Build history of the part. All positions in model axes, mm. A direction names the side the tool comes from. Coordinates: 2 decimals unless noted, no trailing zeros. Order: outer loops, then holes, each group sorted by start corner. A loop starts at its lowest first (then second) coordinate and runs counter-clockwise, first axis right, second up. Notation, with made-up numbers: (3, 84.5) - (37, 84.5) arc R15 ccw to (37, 111.5) - close; hole circle Ø11 at (80, -33.75). An arc over 180 degrees is marked (long way). Return JSON: item names as keys, results as strings.
from build123d import *

# Parameters (mm, degrees)
BOSS_EXTRUDE1_DEPTH = 5
CUT_EXTRUDE1_DEPTH  = 8
CUT_EXTRUDE5_DEPTH  = 3
CUT_EXTRUDE6_DEPTH  = 5
CUT_EXTRUDE7_DEPTH  = 10
CUT_EXTRUDE10_DEPTH = 1


with BuildPart() as part:
    # Sketch1 → Boss-Extrude1 (new body, symmetric)
    with BuildSketch(Plane.XY):
        Polygon((7, -6), (7, 0), (0, 0), (0, -2), (0, -4), (2, -4), (2, -2), (5, -2), (5, -6), align=None)
        Polygon((4, -6), (5, -6), (5, -2), (2, -2), (2, -4), (0, -4), (0, -2), (-1, -2), (-1, -5), (2, -7), (4, -7), align=None)
    extrude(amount=BOSS_EXTRUDE1_DEPTH, both=True)

    # Sketch2 → Cut-Extrude1 (cut)
    with BuildSketch(Plane.XY.offset(5)):
        Polygon((5, -6), (5, -2), (2, -2), (2, -4), (0, -4), (0, -2), (-1, -2), (-1, -5), (2, -7), (4, -7), (4, -6), align=None)
    extrude(amount=-CUT_EXTRUDE1_DEPTH, mode=Mode.SUBTRACT)

    # Sketch4 → Cut-Extrude5 (cut, through all)
    with BuildSketch(Plane.XZ.offset(2)):
        Polygon((5, 5), (0, 0), (0, 5), align=None)
    extrude(amount=-CUT_EXTRUDE5_DEPTH, mode=Mode.SUBTRACT)

    # Sketch5 → Cut-Extrude6 (cut, through all)
    with BuildSketch(Plane.XZ.offset(4)):
        Polygon((2, 2), (0, 0), (0, 5), (2, 5), align=None)
    extrude(amount=-CUT_EXTRUDE6_DEPTH, mode=Mode.SUBTRACT)

    # Sketch9 → Cut-Extrude7 (cut)
    with BuildSketch(Plane(origin=(0, 0, 0), x_dir=(0.596284794, 0.298142397, 0.745355992), z_dir=(-0.666666667, -0.333333333, 0.666666667))):
        Polygon((0, 0), (-2.683281573, -3.577708764), (4.829366967, -9.212195169), (9.390810676, -3.130270225), align=None)
    extrude(amount=CUT_EXTRUDE7_DEPTH, mode=Mode.SUBTRACT)

    # Sketch10 → Cut-Extrude10 (cut)
    with BuildSketch(Plane(origin=(7, 0, 0), x_dir=(0, 0, -1), z_dir=(1, 0, 0))):
        Polygon((-4, -6), (-5, -6), (-5, -3.998994023), align=None)
    extrude(amount=-CUT_EXTRUDE10_DEPTH, mode=Mode.SUBTRACT)


solid = part.part
1. Cut at A-A on z = -3.5. Give the cut face in (x, y), plus the area to 3 significant figures.
Check values:
{"outline": "(-1, -5) - (2, -7) - (4, -7) - (4, -6) - (7, -6) - (7, 0) - (0, 0) - (0, -2) - (-1, -2) - close", "area": "48.0 mm²"}
2. Cut at B-B on x = 4.75. Give the cut face in (y, z).
Check values:
{"outline": "(-6, -5) - (0, -5) - (0, 4.75) - (-2, 3.75) - (-2, -3) - (-6, -3) - close"}
3. Drop flat-ended pins along their axis: pin 1 (3 mm diameter, centred on y = -1.5, z = -1, fed in from -X); pin 2 (0.9 mm diameter, centred on x = 6, z = -1.5, fed in from -Y); pin 3 (1.6 mm diameter, centred on x = 1, z = -2, fed in from -Y). Give the stop position or say it passes through.
Check values:
{"pin 1": "x = 0", "pin 2": "y = -6", "pin 3": "y = -4"}
4. Mould opens along X. For faces 5 (the flat face through (2, -3, -1)), 6 (the flat face through (6, -6, -1)), 7 (the flat face through (3.86, -1.7, 3.01)) say: pulls with the +X half, pulls with the -X half, needs draft (parallel to the pull), parting line crosses it, or undercut.
Check values:
{"face 5": "undercut", "face 6": "needs draft", "face 7": "pulls with the -X half"}
5. Cut at D-D on z = 0.25. Give the cut face in (x, y), plus the area to 3 significant figures.
Check values:
{"outline": "(0.25, 0) - (2, -3.5) - (2, -2) - (5, -2) - (5, -6) - (7, -6) - (7, 0) - close", "area": "21.1 mm²"}
6. Tool access for faces 1 (the flat face through (1, -4, -2)), 2 (the flat face through (5, -4, 0)), 3 (the flat face through (4, -6.5, -4)), 4 (the flat face through (3, -7, -4)): list every direction of +Z, -Z, +X, -X, +Y, -Y with a clear straight run to the whole face (end or side of a thin tool).
Check values:
{"face 1": "+Z, -X, -Y", "face 2": "+Z, -Y", "face 3": "+Z, -Z, +X, -Y", "face 4": "+Z, -Z, +X, -X, -Y"}
7. Probe L1, parallel to Y at x = 4, z = -1.25; L2, parallel to X at y = -1, z = -1.5; L3, parallel to X at y = -5.25, z = 1. List the from-to ranges inside material, lowest first.
Check values:
{"L1": "-2 to 0", "L2": "0 to 7", "L3": "5 to 7"}
